For this review, take the finished solid that the model builds, in its own axes (mm). Face numbers are marked on the shaded views. A direction names the side the tool comes from. Round coordinates to 2 decimals unless told otherwise and drop trailing zeros. Order: outer loops, then holes, each group sorted by start corner. A loop starts at its lowest first (then second) coordinate and runs counter-clockwise, first axis right, second up.
from build123d import *

# Parameters (mm, degrees)
SKETCH2_R           = 6
SKETCH2_R_2         = 5
BOSS_EXTRUDE1_DEPTH = 4
SKETCH3_R           = 12
BOSS_EXTRUDE2_DEPTH = 9
BOSS_EXTRUDE3_START = 30
SKETCH4_R           = 6
BOSS_EXTRUDE3_DEPTH = 30
BOSS_EXTRUDE4_START = -8
BOSS_EXTRUDE4_DEPTH = 8
CUT_EXTRUDE2_DEPTH  = 10


with BuildPart() as part:
    # Sketch1 → Revolve1 (revolve)
    with BuildSketch(Plane.XY):
        with BuildLine():
            Line((-19, 0), (-17, 0))
            Line((-17, 0), (-17, 21))
            ThreePointArc((-17, 21), (-16.121320344, 23.121320344), (-14, 24))
            Line((-14, 24), (0, 24))
            Line((0, 24), (0, 26))
            Line((0, 26), (-16, 26))
            ThreePointArc((-16, 26), (-18.121320344, 25.121320344), (-19, 23))
            Line((-19, 23), (-19, 0))
        make_face()
    revolve(axis=Axis((0, 0, 0), (-1, 0, 0)))

    # Sketch2 → Boss-Extrude1 (add)
    with BuildSketch(Plane(origin=(-17, 0, 0), x_dir=(0, 0, -1), z_dir=(1, 0, 0))):
        with Locations(Location((0, 0, 0), (0, 0, 90))):
            Circle(SKETCH2_R)
        with Locations(Location((0, 0, 0), (0, 0, 90))):
            Circle(SKETCH2_R_2, mode=Mode.SUBTRACT)
    extrude(amount=BOSS_EXTRUDE1_DEPTH)

    # Sketch3 → Boss-Extrude2 (add)
    with BuildSketch(Plane.ZY.offset(19)):
        with Locations(Location((0, 0, 0), (0, 0, 270))):
            Circle(SKETCH3_R)
    extrude(amount=BOSS_EXTRUDE2_DEPTH)

    # Sketch4 → Boss-Extrude3 (add)
    with BuildSketch(Plane.ZY.offset(28).offset(BOSS_EXTRUDE3_START)):
        with Locations(Location((0, 0, 0), (0, 0, 90))):
            Circle(SKETCH4_R)
    extrude(amount=-BOSS_EXTRUDE3_DEPTH)

    # Sketch5 → Boss-Extrude4 (add)
    with BuildSketch(Plane(origin=(0, 0, 0), x_dir=(0, 0, -1), z_dir=(1, 0, 0)).offset(BOSS_EXTRUDE4_START)):
        with BuildLine():
            Line((0, 26), (0, 27))
            ThreePointArc((0, 27), (4.688500797, 26.589809331), (9.23454387, 25.371700761))
            Line((9.23454387, 25.371700761), (8.892523726, 24.43200814))
            ThreePointArc((8.892523726, 24.43200814), (4.514852619, 25.605001578), (0, 26))
        make_face()
        with BuildLine():
            Line((22.516660498, 13), (23.382685902, 13.5))
            ThreePointArc((23.382685902, 13.5), (25.371700761, 9.23454387), (26.589809331, 4.688500797))
            Line((26.589809331, 4.688500797), (25.605001578, 4.514852619))
            ThreePointArc((25.605001578, 4.514852619), (24.43200814, 8.892523726), (22.516660498, 13))
        make_face()
        with BuildLine():
            Line((22.516660498, -13), (23.382685902, -13.5))
            ThreePointArc((23.382685902, -13.5), (20.683199964, -17.355265462), (17.355265462, -20.683199964))
            Line((17.355265462, -20.683199964), (16.712477852, -19.917155521))
            ThreePointArc((16.712477852, -19.917155521), (19.917155521, -16.712477852), (22.516660498, -13))
        make_face()
        with BuildLine():
            Line((0, -26), (0, -27))
            ThreePointArc((0, -27), (-4.688500797, -26.589809331), (-9.23454387, -25.371700761))
            Line((-9.23454387, -25.371700761), (-8.892523726, -24.43200814))
            ThreePointArc((-8.892523726, -24.43200814), (-4.514852619, -25.605001578), (0, -26))
        make_face()
        with BuildLine():
            Line((-22.516660498, -13), (-23.382685902, -13.5))
            ThreePointArc((-23.382685902, -13.5), (-25.371700761, -9.23454387), (-26.589809331, -4.688500797))
            Line((-26.589809331, -4.688500797), (-25.605001578, -4.514852619))
            ThreePointArc((-25.605001578, -4.514852619), (-24.43200814, -8.892523726), (-22.516660498, -13))
        make_face()
        with BuildLine():
            Line((-22.516660498, 13), (-23.382685902, 13.5))
            ThreePointArc((-23.382685902, 13.5), (-20.683199964, 17.355265462), (-17.355265462, 20.683199964))
            Line((-17.355265462, 20.683199964), (-16.712477852, 19.917155521))
            ThreePointArc((-16.712477852, 19.917155521), (-19.917155521, 16.712477852), (-22.516660498, 13))
        make_face()
    extrude(amount=BOSS_EXTRUDE4_DEPTH)

    # Sketch6 → Cut-Extrude2 (cut)
    with BuildSketch(Plane.ZY.offset(58)):
        with BuildLine():
            ThreePointArc((-1.775009671, 4.135134903), (-1.847979553, 4.927336232), (-1.805897134, 5.721777306))
            ThreePointArc((-1.805897134, 5.721777306), (-2.788339032, 5.312736154), (-3.683063909, 4.736564181))
            ThreePointArc((-3.683063909, 4.736564181), (-3.005346184, 4.319903366), (-2.394828889, 3.809828683))
            ThreePointArc((-2.394828889, 3.809828683), (-1.967355774, 3.748483247), (-1.775009671, 4.135134903))
        make_face()
        with BuildLine():
            ThreePointArc((-3.493386018, 2.836591992), (-3.926151954, 3.504140637), (-4.258084999, 4.227139948))
            ThreePointArc((-4.258084999, 4.227139948), (-4.937903195, 3.40838848), (-5.462382262, 2.482414153))
            ThreePointArc((-5.462382262, 2.482414153), (-4.668661083, 2.428430454), (-3.891031341, 2.260503286))
            ThreePointArc((-3.891031341, 2.260503286), (-3.484014049, 2.404841262), (-3.493386018, 2.836591992))
        make_face()
        with BuildLine():
            ThreePointArc((-4.411469728, 0.88822004), (-5.104890258, 1.278188652), (-5.734796905, 1.764115771))
            ThreePointArc((-5.734796905, 1.764115771), (-5.956253245, 0.723220082), (-5.990334668, -0.340427042))
            ThreePointArc((-5.990334668, -0.340427042), (-5.262441991, -0.019366609), (-4.495845404, 0.193323828))
            ThreePointArc((-4.495845404, 0.193323828), (-4.202526693, 0.510279126), (-4.411469728, 0.88822004))
        make_face()
        with BuildLine():
            ThreePointArc((-4.318938887, -1.263632419), (-5.114159724, -1.24058095), (-5.897735953, -1.103046069))
            ThreePointArc((-5.897735953, -1.103046069), (-5.610097456, -2.127629322), (-5.145973592, -3.085280504))
            ThreePointArc((-5.145973592, -3.085280504), (-4.650660859, -2.462727016), (-4.070715466, -1.918143789))
            ThreePointArc((-4.070715466, -1.918143789), (-3.958291117, -1.501181809), (-4.318938887, -1.263632419))
        make_face()
        with BuildLine():
            ThreePointArc((-3.236991196, -3.126001919), (-3.95183683, -3.475148407), (-4.709574769, -3.717513349))
            ThreePointArc((-4.709574769, -3.717513349), (-3.978735949, -4.491064489), (-3.122731983, -5.123333384))
            ThreePointArc((-3.122731983, -5.123333384), (-2.97346937, -4.341906342), (-2.713033672, -3.59018778))
            ThreePointArc((-2.713033672, -3.59018778), (-2.807258749, -3.168740082), (-3.236991196, -3.126001919))
        make_face()
        with BuildLine():
            ThreePointArc((-1.413487832, -4.272242052), (-1.884195742, -4.913601244), (-2.442506762, -5.480343121))
            ThreePointArc((-2.442506762, -5.480343121), (-1.435893986, -5.825650905), (-0.384110109, -5.987692329))
            ThreePointArc((-0.384110109, -5.987692329), (-0.615091883, -5.226407251), (-0.73382856, -4.439763017))
            ThreePointArc((-0.73382856, -4.439763017), (-1.013117233, -4.11037819), (-1.413487832, -4.272242052))
        make_face()
        with BuildLine():
            ThreePointArc((0.384110109, -5.987692329), (1.435893986, -5.825650905), (2.442506762, -5.480343121))
            ThreePointArc((2.442506762, -5.480343121), (1.884195742, -4.913601244), (1.413487832, -4.272242052))
            ThreePointArc((1.413487832, -4.272242052), (1.013117233, -4.11037819), (0.73382856, -4.439763017))
            ThreePointArc((0.73382856, -4.439763017), (0.615091883, -5.226407251), (0.384110109, -5.987692329))
        make_face()
        with BuildLine():
            ThreePointArc((3.122731983, -5.123333384), (3.978735949, -4.491064489), (4.709574769, -3.717513349))
            ThreePointArc((4.709574769, -3.717513349), (3.95183683, -3.475148407), (3.236991196, -3.126001919))
            ThreePointArc((3.236991196, -3.126001919), (2.807258749, -3.168740082), (2.713033672, -3.59018778))
            ThreePointArc((2.713033672, -3.59018778), (2.97346937, -4.341906342), (3.122731983, -5.123333384))
        make_face()
        with BuildLine():
            ThreePointArc((5.145973592, -3.085280504), (5.610097456, -2.127629322), (5.897735953, -1.103046069))
            ThreePointArc((5.897735953, -1.103046069), (5.114159724, -1.24058095), (4.318938887, -1.263632419))
            ThreePointArc((4.318938887, -1.263632419), (3.958291117, -1.501181809), (4.070715466, -1.918143789))
            ThreePointArc((4.070715466, -1.918143789), (4.650660859, -2.462727016), (5.145973592, -3.085280504))
        make_face()
        with BuildLine():
            ThreePointArc((6, 0), (5.933328806, 0.891969329), (5.734796905, 1.764115771))
            ThreePointArc((5.734796905, 1.764115771), (5.104890258, 1.278188652), (4.411469728, 0.88822004))
            ThreePointArc((4.411469728, 0.88822004), (4.202526693, 0.510279126), (4.495845404, 0.193323828))
            ThreePointArc((4.495845404, 0.193323828), (5.262441991, -0.019366609), (5.990334668, -0.340427042))
            ThreePointArc((5.990334668, -0.340427042), (5.99758318, -0.170282111), (6, 0))
        make_face()
        with BuildLine():
            ThreePointArc((5.462382262, 2.482414153), (4.937903195, 3.40838848), (4.258084999, 4.227139948))
            ThreePointArc((4.258084999, 4.227139948), (3.926151954, 3.504140637), (3.493386018, 2.836591992))
            ThreePointArc((3.493386018, 2.836591992), (3.484014049, 2.404841262), (3.891031341, 2.260503286))
            ThreePointArc((3.891031341, 2.260503286), (4.668661083, 2.428430454), (5.462382262, 2.482414153))
        make_face()
        with BuildLine():
            ThreePointArc((3.683063909, 4.736564181), (2.788339032, 5.312736154), (1.805897134, 5.721777306))
            ThreePointArc((1.805897134, 5.721777306), (1.847979553, 4.927336232), (1.775009671, 4.135134903))
            ThreePointArc((1.775009671, 4.135134903), (1.967355774, 3.748483247), (2.394828889, 3.809828683))
            ThreePointArc((2.394828889, 3.809828683), (3.005346184, 4.319903366), (3.683063909, 4.736564181))
        make_face()
        with BuildLine():
            ThreePointArc((1.06, 5.905624438), (0, 6), (-1.06, 5.905624438))
            ThreePointArc((-1.06, 5.905624438), (-0.653542693, 5.221738477), (-0.35, 4.486368242))
            ThreePointArc((-0.35, 4.486368242), (0, 4.233392894), (0.35, 4.486368242))
            ThreePointArc((0.35, 4.486368242), (0.653542693, 5.221738477), (1.06, 5.905624438))
        make_face()
    extrude(amount=-CUT_EXTRUDE2_DEPTH, mode=Mode.SUBTRACT)


solid = part.part
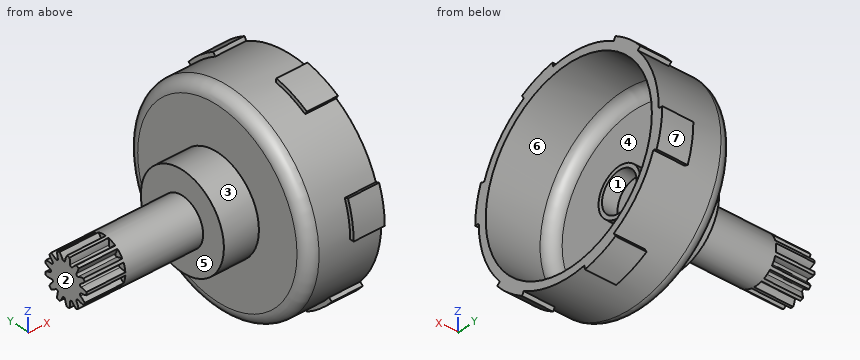
(1) Draft analysis for pull direction Y (two halves, no side actions). For the marked faces 1, 2, 3 and 4, state which applies: pulls with the +Y half, pulls with the -Y half, needs draft (parallel to the pull), parting line crosses it, or undercut.
(2) Clearance check with flat-ended pins moving along their axes: P1, Ø3, axis at y = -18, z = 6, coming from the +X side; P2, Ø1.5, axis at y = 1.5, z = -21, coming from the -X side; P3, Ø8, axis at y = -11.5, z = -8, coming from the -X side. State where each tip first meets the part, or that it passes through.
(3) Wall thickness on L1, parallel to Z at x = -10, y = 0; L2, parallel to Z at x = -5, y = -20.5; L3, parallel to X at y = -17.5, z = -1: over which ranges is each line inside the solid? List them lowest first.
(4) Tool access review of the marked faces 5, 6 and 7: name each direction out of +Z, -Z, +X, -X, +Y, -Y from which nothing blocks a thin tool from reaching the whole face with its end or side.
(5) Add section B-B on x = -47. Give the boundary of the cut face in (y, z).
(6) Add section A-A on x = -7. Give the boundary of the cut face in (y, z) (1 decimal).
Here are the results:
1. face 1: undercut
1. face 2: needs draft
1. face 3: parting line crosses it
1. face 4: undercut
2. P1: stops at x = -17
2. P2: stops at x = -19
2. P3: stops at x = -28
3. L1: z = -26 to -24, 24 to 26
3. L2: z = -17.57 to -17.2, -15.99 to -12.48, 12.48 to 15.99
3. L3: x = -19 to -17
4. face 5: -X
4. face 6: +X
4. face 7: -Z, +X, -X, +Y
5. outline: circle Ø12 at (0, 0)
6. outline: (-27, 0) - (-26, 0) arc R26 ccw to (-19.9, -16.7) - (-20.7, -17.4) arc R27 ccw to (-13.5, -23.4) - (-13, -22.5) arc R26 ccw to (4.5, -25.6) - (4.7, -26.6) arc R27 ccw to (13.5, -23.4) - (13, -22.5) arc R26 ccw to (24.4, -8.9) - (25.4, -9.2) arc R27 ccw to (27, 0) - (26, 0) arc R26 ccw to (19.9, 16.7) - (20.7, 17.4) arc R27 ccw to (13.5, 23.4) - (13, 22.5) arc R26 ccw to (-4.5, 25.6) - (-4.7, 26.6) arc R27 ccw to (-13.5, 23.4) - (-13, 22.5) arc R26 ccw to (-24.4, 8.9) - (-25.4, 9.2) arc R27 ccw to start; hole circle Ø48 at (0, 0)
